Geometry check sheet. Reference: the model listing, model coordinates, mm. A direction names the side the tool comes from. Coordinates: 2 decimals unless noted, no trailing zeros. Order: outer loops, then holes, each group sorted by start corner. A loop starts at its lowest first (then second) coordinate and runs counter-clockwise, first axis right, second up.
```python
from build123d import *

# Parameters (mm, degrees)
F1_DEPTH = 12.7


with BuildPart() as f1:
    # F0 (on Front) → F1 (new body)
    with BuildSketch(Plane.XZ):
        Polygon((-34.601895, 47.571581), (-56.804623, 47.571581), (-56.804623, -9.578419), (-33.77184, -9.578419), (-33.77184, -0.624114), (-29.897187, -9.578419), (-11.936555, -9.578419), (-11.936555, 47.571581), (-30.986555, 47.571581), (-30.986555, 35.822231), align=None)
        Polygon((-36.94684, -6.403419), (-53.629623, -6.403419), (-53.629623, 44.396581), (-36.94684, 44.396581), (-27.811555, 14.708183), (-27.811555, 44.396581), (-15.111555, 44.396581), (-15.111555, -6.403419), (-27.811555, -6.403419), (-36.94684, 14.708183), align=None, mode=Mode.SUBTRACT)
    extrude(amount=F1_DEPTH)


solid = f1.part
```
Item 1: Sectioned sample at D-D (z = 29.5). Record the cut outline in (x, y), and give its area (3 significant figures).
Item 2: Depth check by flat-ended pin: P1, Ø10, axis at x = -36.5, z = 20.5, coming from the +Y side. Enter the tip coordinate at first touch or a pass-through.
Item 3: Sectioned sample at B-B (z = 40.5). Record the cut outline in (x, y), and give its area (3 significant figures).
Item 4: Thickness scan on line 1 along Z through (x, y) = (-21.5, -6.5); line 2 along X through (y, z) = (-11, 26.5); line 3 along X through (y, z) = (-4.25, 37). Record the ranges inside material, lowest first.
Item 5: Sectioned sample at C-C (x = -19). Record the cut outline in (y, z), and give its area (3 significant figures).
Item 6: Tool access check on faces 1 (the face through (-30, -12.7, 26)), 2 (the face through (-32.315, -6.261, 4.005)). Record the directions out of +Z, -Z, +X, -X, +Y, -Y that give a thin tool (end or side, any length) a straight path to the whole face; none if there is none.
Item 7: Sectioned sample at A-A (y = -10). Record the cut outline in (x, z).
Item 8: Release check for a two-part mould opening along Z. For faces 3 (the face through (-46, -6, 47.572)), 4 (the face through (-11.937, -6, 19)), 5 (the face through (-32.443, -6.261, 29.76)) record: pulls with the +Z half, pulls with the -Z half, needs draft (parallel to the pull), parting line crosses it, or undercut.
Geometry check:
1. outline: (-56.8, -12.7) - (-53.63, -12.7) - (-53.63, 0) - (-56.8, 0) - close; (-32.36, -12.7) - (-27.81, -12.7) - (-27.81, 0) - (-32.36, 0) - close; (-15.11, -12.7) - (-11.94, -12.7) - (-11.94, 0) - (-15.11, 0) - close
1. area: 138 mm2
2. P1: passes through
3. outline: (-56.8, -12.7) - (-53.63, -12.7) - (-53.63, 0) - (-56.8, 0) - close; (-35.75, -12.7) - (-32.43, -12.7) - (-32.43, 0) - (-35.75, 0) - close; (-30.99, -12.7) - (-27.81, -12.7) - (-27.81, 0) - (-30.99, 0) - close; (-15.11, -12.7) - (-11.94, -12.7) - (-11.94, 0) - (-15.11, 0) - close
3. area: 163 mm2
4. line 1: z = -9.58 to -6.4, 44.4 to 47.57
4. line 2: x = -56.8 to -53.63, -31.44 to -27.81, -15.11 to -11.94
4. line 3: x = -56.8 to -53.63, -34.67 to -31.35, -30.99 to -27.81, -15.11 to -11.94
5. outline: (-12.7, -9.58) - (0, -9.58) - (0, -6.4) - (-12.7, -6.4) - close; (-12.7, 44.4) - (0, 44.4) - (0, 47.57) - (-12.7, 47.57) - close
5. area: 80.6 mm2
6. face 1: +Z, -Z, +X, -X, -Y
6. face 2: +Y, -Y
7. outline: (-56.8, -9.58) - (-33.77, -9.58) - (-33.77, -0.62) - (-29.9, -9.58) - (-11.94, -9.58) - (-11.94, 47.57) - (-30.99, 47.57) - (-30.99, 35.82) - (-34.6, 47.57) - (-56.8, 47.57) - close; hole (-53.63, -6.4) - (-36.95, -6.4) - (-36.95, 14.71) - (-27.81, -6.4) - (-15.11, -6.4) - (-15.11, 44.4) - (-27.81, 44.4) - (-27.81, 14.71) - (-36.95, 44.4) - (-53.63, 44.4) - close
8. face 3: pulls with the +Z half
8. face 4: needs draft
8. face 5: undercut
